from build123d import *

# Parameters (mm, degrees)
EXTRUDE_1_DEPTH     = 60
SKETCH_2_R          = 5.75
CUT_EXTRUDE_1_DEPTH = 2


with BuildPart() as part:
    # 草图1 → 凸台-拉伸1 (new body)
    with BuildSketch(Plane(origin=(0, 0, 0), x_dir=(1, 0, 0), z_dir=(0, 1, 0))):
        Polygon((0, 0), (80, 30), (80, 0), align=None)
    extrude(amount=EXTRUDE_1_DEPTH)

    # 草图2 → 切除-拉伸1 (cut)
    with BuildSketch(Plane.XY):
        with Locations((70, 50)):
            Circle(SKETCH_2_R)
        with Locations((70, 30)):
            Circle(SKETCH_2_R)
        with Locations((70, 10)):
            Circle(SKETCH_2_R)
    extrude(amount=-CUT_EXTRUDE_1_DEPTH, mode=Mode.SUBTRACT)


solid = part.part
Source: CAD feature listing. Evaluate the final solid. Frame: model axes, mm. A direction names the side the tool comes from. Coordinates: 2 decimals unless noted, no trailing zeros. Loops run counter-clockwise (first coordinate to the right, second up) from the corner with the lowest first, then second, coordinate; pieces in that order, holes last. Notation, with made-up numbers: (61, 78.25) - (79, 78.25) arc R17 cw to (79, 85.25) - close; hole circle Ø4 at (79, -22). An arc over 180 degrees is marked (long way). One line per item, written item: value. Start each with the question number.
1. Set-up query: faces 1 (the flat face through (58, 60, -9)), 2 (the cylindrical face through (65.44, 26.5, -0.99)). Return all of +Z, -Z, +X, -X, +Y, -Y with unobstructed straight access to the full face (end or side cutting, diameter ignored); none if empty.
2. Mould query, pull axis X, two halves, no side actions, for faces 3 (the flat face through (39.44, 29.58, -14.79)), 4 (the flat face through (41, 30, 0)), 5 (the flat face through (70, 50, -2)), 6 (the flat face through (80, 30, -15)). Classes: pulls with the +X half, pulls with the -X half, needs draft (parallel to the pull), parting line crosses it, or undercut.
3. Section B-B (x = 70). Return the cut outline in (y, z).
4. Section A-A (y = 30). Return the cut outline in (x, z), and give its area (3 significant figures).
5. Section D-D (y = 46). Return the cut outline in (x, z), and give its area (3 significant figures).
6. Contact query for flat-ended pins moving along their axis: P1, Ø3.5, axis at x = 69.5, y = 51, coming from the +Z side; P2, Ø8, axis at x = 45, y = 14.5, coming from the -Z side (3 decimals). Output: stop coordinate, or through.
7. Section C-C (z = -3.75). Return the cut outline in (x, y), and give its area (3 significant figures).
8. Ray query, L1, parallel to Y at x = 70, z = -0.5; L2, parallel to Z at x = 67, y = 53 (3 decimals); L3, parallel to Z at x = 5.5, y = 46. Return the intervals inside material, ascending.
Verdict:
1. face 1: +Z, -Z, +X, -X, +Y
1. face 2: +Z
2. face 3: pulls with the -X half
2. face 4: needs draft
2. face 5: undercut
2. face 6: pulls with the +X half
3. outline: (0, -26.25) - (60, -26.25) - (60, 0) - (55.75, 0) - (55.75, -2) - (44.25, -2) - (44.25, 0) - (35.75, 0) - (35.75, -2) - (24.25, -2) - (24.25, 0) - (15.75, 0) - (15.75, -2) - (4.25, -2) - (4.25, 0) - (0, 0) - close
4. outline: (0, 0) - (80, -30) - (80, 0) - (75.75, 0) - (75.75, -2) - (64.25, -2) - (64.25, 0) - close
4. area: 1,180 mm2
5. outline: (0, 0) - (80, -30) - (80, 0) - (74.13, 0) - (74.13, -2) - (65.87, -2) - (65.87, 0) - close
5. area: 1,180 mm2
6. P1: stops at z = -2
6. P2: stops at z = -18.375
7. outline: (10, 0) - (80, 0) - (80, 60) - (10, 60) - close
7. area: 4,200 mm2
8. L1: y = 0 to 4.25, 15.75 to 24.25, 35.75 to 44.25, 55.75 to 60
8. L2: z = -25.125 to -2
8. L3: z = -2.06 to 0
